Work out the finished part from the listing and answer in its coordinate system (mm). A direction names the side the tool comes from. Give positions to 0.01 mm unless a question says otherwise; leave off trailing zeros. Loops run counter-clockwise (first coordinate to the right, second up) from the corner with the lowest first, then second, coordinate; pieces in that order, holes last.
from build123d import *

# Parameters (mm, degrees)
F0_W     = 25.4
F0_H     = 2.54
F1_DEPTH = 25.4
F2_R     = 3.175
F3_DEPTH = 25.4
F4_W     = 12.7
F4_H     = 4.445
F5_DEPTH = 9.525
F6_W     = 12.7
F6_H     = 2.54
F7_DEPTH = 3.175
F8_W     = 0.635
F8_H     = 3.175
F9_DEPTH = 0.254


with BuildPart() as f1:
    # F0 (on Right) → F1 (new body)
    with BuildSketch(Plane.YZ):
        Rectangle(F0_W, F0_H)
    extrude(amount=F1_DEPTH)

    # F2 (on face) → F3 (cut)
    with BuildSketch(Plane.XY.offset(1.27)):
        with Locations((12.7, 0)):
            Circle(F2_R)
    extrude(amount=-F3_DEPTH, mode=Mode.SUBTRACT)

    # F4 (on face) → F5 (join)
    with BuildSketch(Plane(origin=(0, 0, -1.27), x_dir=(1, 0, 0), z_dir=(0, 0, -1))):
        with Locations((13.610998, 6.782856)):
            Rectangle(F4_W, F4_H)
    extrude(amount=F5_DEPTH)

    # F6 (on face) → F7 (cut)
    with BuildSketch(Plane.XZ.offset(9.005356)):
        with Locations((13.610998, -7.3025)):
            Rectangle(F6_W, F6_H)
    extrude(amount=-F7_DEPTH, mode=Mode.SUBTRACT)

    # F8 (on face) → F9 (join)
    with BuildSketch(Plane.XY.offset(-8.5725)):
        with Locations((8.873898, -7.417856)):
            Rectangle(F8_W, F8_H)
        with Locations((7.578498, -7.417856)):
            Rectangle(F8_W, F8_H)
        with Locations((10.169298, -7.417856)):
            Rectangle(F8_W, F8_H)
        with Locations((11.464698, -7.417856)):
            Rectangle(F8_W, F8_H)
        with Locations((12.760098, -7.417856)):
            Rectangle(F8_W, F8_H)
        with Locations((14.055498, -7.417856)):
            Rectangle(F8_W, F8_H)
        with Locations((15.350898, -7.417856)):
            Rectangle(F8_W, F8_H)
        with Locations((16.646298, -7.417856)):
            Rectangle(F8_W, F8_H)
        with Locations((17.941698, -7.417856)):
            Rectangle(F8_W, F8_H)
        with Locations((19.237098, -7.417856)):
            Rectangle(F8_W, F8_H)
    extrude(amount=F9_DEPTH)


solid = f1.part
Item 1: Find section C-C, the plane x = 4. Write down the section's boundary in (y, z), plus the area to 3 significant figures.
Item 2: Determine the mould class of faces 1 (the face through (14, -5.83, -7)), 2 (the face through (14, -7, -10.795)), 3 (the face through (14, -9.005, -10)) for opening direction Z: released by +Z, released by -Z, zero draft, split by the parting line, or undercut.
Item 3: Find section A-A, the plane y = 0. Write down the section's boundary in (x, z) (3 decimals).
Item 4: For faces 4 (the face through (19.961, -7, -5)), 5 (the face through (14, -7, -6.033)), 6 (the face through (14, -4.56, -6)), 7 (the face through (7.261, -7, -5)), determine the directions among +Z, -Z, +X, -X, +Y, -Y from which every point of the face is accessible in a straight line to the end or side of a thin tool.
Item 5: Find section B-B, the plane z = -0.5. Write down the section's boundary in (x, y) (3 decimals), plus the area to 3 significant figures.
Item 6: Find section D-D, the plane y = 4. Write down the section's boundary in (x, z).
Item 7: Consider line 1 (Y direction, x = 12.7, z = 0.6) (3 decimals); line 2 (Z direction, x = 15.5, y = 11.5); line 3 (Z direction, x = 15.5, y = -6) (1 decimal). Determine where each line is inside the solid, lowest interval first.
Item 8: Flat-ended cylindrical pins translate along their axes: pin 1 Ø1.5 at (x, y) = (6.5, -1) entering from -Z; pin 2 Ø0.7 at (x, z) = (12, -9.5) entering from -Y; pin 3 Ø1.3 at (y, z) = (-7.5, -4.5) entering from -X; pin 4 Ø6 at (y, z) = (9, -3) entering from +X. Find the tip coordinate at first contact, or state that the pin passes through.
Ans:
1. outline: (-12.7, -1.27) - (12.7, -1.27) - (12.7, 1.27) - (-12.7, 1.27) - close
1. area: 64.5 mm2
2. face 1: undercut
2. face 2: released by -Z
2. face 3: zero draft
3. outline: (0, -1.27) - (9.525, -1.27) - (9.525, 1.27) - (0, 1.27) - close; (15.875, -1.27) - (25.4, -1.27) - (25.4, 1.27) - (15.875, 1.27) - close
4. face 4: -Z, +X, +Y, -Y
4. face 5: +X, -X, -Y
4. face 6: -Z, +X, -X, +Y
4. face 7: -Z, -X, +Y, -Y
5. outline: (0, -12.7) - (25.4, -12.7) - (25.4, 12.7) - (0, 12.7) - close; hole circle Ø6.35 at (12.7, 0)
5. area: 613 mm2
6. outline: (0, -1.27) - (25.4, -1.27) - (25.4, 1.27) - (0, 1.27) - close
7. line 1: y = -12.7 to -3.175, 3.175 to 12.7
7. line 2: z = -1.27 to 1.27
7. line 3: z = -10.8 to -8.3, -6 to 1.3
8. pin 1: stops at z = -1.27
8. pin 2: stops at y = -9.01
8. pin 3: stops at x = 7.26
8. pin 4: stops at x = 25.4
